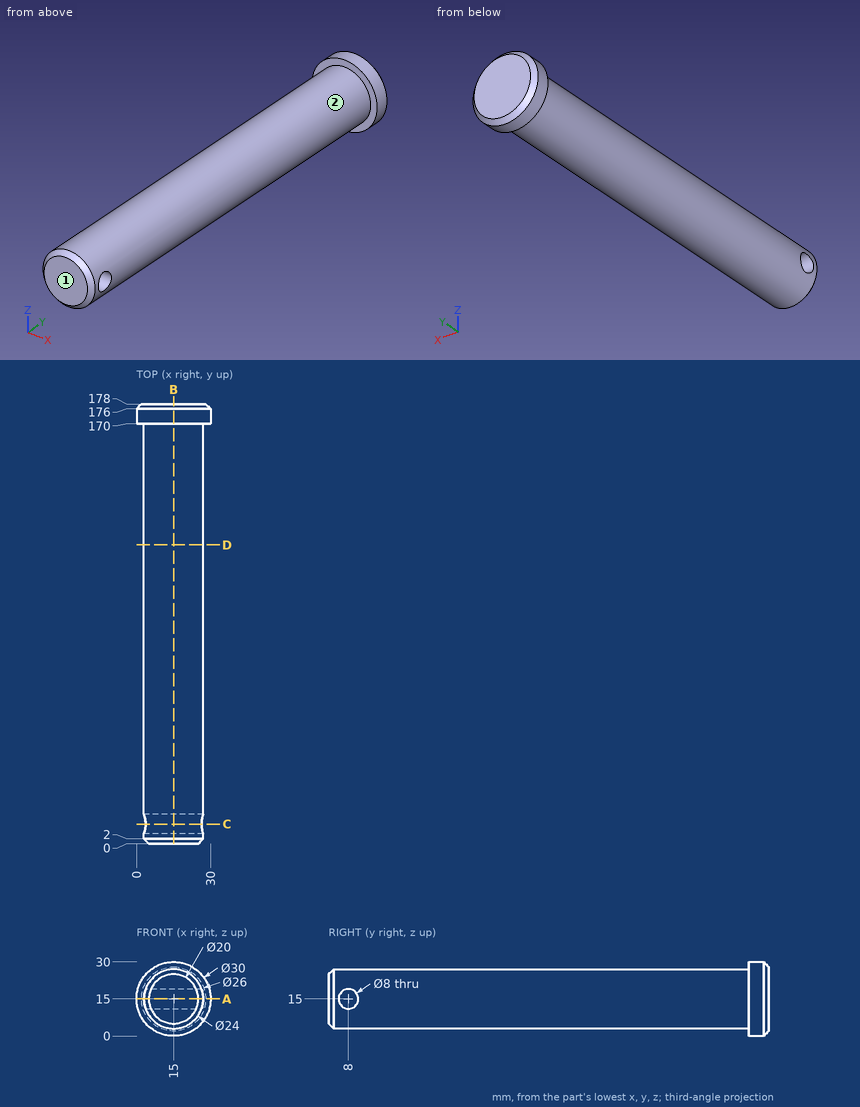
The figure shows three views and two pictorial views of one solid part (mm, origin at its lowest corner). Answer the questions. Round coordinates to 2 decimals unless told otherwise and drop trailing zeros. Write each loop counter-clockwise with the first axis right and the second up, starting at its lowest first coordinate (ties: lowest second). Pieces come first, ordered by that corner, then holes. Notation, with made-up numbers: (11, 57) - (60, 57) arc R19 ccw to (60, 63) - close; hole circle Ø5 at (3.25, 81.25). An arc over 180 degrees is marked (long way). Use one line per item in the form item = value. Start each with the question number.
Item 1: Flat-ended cylindrical pins translate along their axes: pin 1 Ø4 at (y, z) = (57, 26) entering from +X; pin 2 Ø1 at (x, y) = (5.5, 112) entering from -Z; pin 3 Ø1.5 at (x, y) = (7, 78.5) entering from +Z; pin 4 Ø5 at (y, z) = (8, 15) entering from -X. Find the tip coordinate at first contact, or state that the pin passes through.
Item 2: A cutting plane is placed at C-C (y = 8). Write down the section's boundary in (x, z).
Item 3: Determine the mould class of the marked faces 1 and 2 for opening direction X: +X half, -X half, draft (parallel to the pull), parting line (faces both ways), or undercut.
Item 4: Find the intervals of material crossed by line 1 (Y direction, x = 12.5, z = 15); line 2 (Y direction, x = 23, z = 15.75); line 3 (Z direction, x = 19, y = 8), in increasing order. Write a range as [from, to].
Item 5: A cutting plane is placed at D-D (y = 121). Write down the section's boundary in (x, z).
Item 6: A cutting plane is placed at B-B (x = 15). Write down the section's boundary in (y, z).
Item 7: A cutting plane is placed at A-A (z = 15). Write down the section's boundary in (x, y).
The answers:
q1.pin_1 = 22.94
q1.pin_2 = 7.06
q1.pin_3 = 24.56
q1.pin_4 = through
q2.outline = (3.69, 11) arc R12 ccw to (26.31, 11) - close; (3.69, 19) - (26.31, 19) arc R12 ccw to start
q3.face_1 = draft
q3.face_2 = parting line
q4.line_1 = [0, 4], [12, 178]
q4.line_2 = [0, 4.07], [11.93, 178]
q4.line_3 = [3.69, 11], [19, 26.31]
q5.outline = circle Ø24 at (15, 15)
q6.outline = (0, 5) - (2, 3) - (170, 3) - (170, 0) - (176, 0) - (178, 2) - (178, 28) - (176, 30) - (170, 30) - (170, 27) - (2, 27) - (0, 25) - close; hole circle Ø8 at (8, 15)
q7.outline = (0, 170) - (3, 170) - (3, 12) - (27, 12) - (27, 170) - (30, 170) - (30, 176) - (28, 178) - (2, 178) - (0, 176) - close; (3, 2) - (5, 0) - (25, 0) - (27, 2) - (27, 4) - (3, 4) - close
